from build123d import *

# Parameters (mm, degrees)
F1_W     = 279.4
F1_H     = 127
F1_W_2   = 254
F1_H_2   = 101.6
F3_DEPTH = 3.175
F2_W     = 285.75
F2_H     = 133.35
F2_W_2   = 279.4
F2_H_2   = 127
F6_DEPTH = 25.4
F7_W     = 254
F7_H     = 101.6
F7_W_2   = 247.65
F7_H_2   = 95.25
F8_DEPTH = 25.4


with BuildPart() as f3:
    # F1 (on Top) → F3 (new body)
    with BuildSketch(Plane.XY):
        Rectangle(F1_W, F1_H)
        Rectangle(F1_W_2, F1_H_2, mode=Mode.SUBTRACT)
    extrude(amount=F3_DEPTH)

    # F2 (on face) → F6 (join)
    with BuildSketch(Plane.XY):
        Rectangle(F2_W, F2_H)
        Rectangle(F2_W_2, F2_H_2, mode=Mode.SUBTRACT)
    extrude(amount=F6_DEPTH)

    # F7 (on face) → F8 (join)
    with BuildSketch(Plane.XY):
        Rectangle(F7_W, F7_H)
        Rectangle(F7_W_2, F7_H_2, mode=Mode.SUBTRACT)
    extrude(amount=F8_DEPTH)


solid = f3.part
Check sheet for the modelled part. Datum: model origin and axes. Units: mm. A direction names the side the tool comes from. Coordinates: 2 decimals unless noted, no trailing zeros. Loops run counter-clockwise (first coordinate to the right, second up) from the corner with the lowest first, then second, coordinate; pieces in that order, holes last. Notation, with made-up numbers: (23.25, 72) -> (44.25, 72) arc R18 cw to (44.25, 88) -> close; hole circle Ø1 at (-33.5, 81). An arc over 180 degrees is marked (long way). Write item = value, one per line. Start each with the question number.
1. Draft check along Y on faces 4 (the flat face through (-127, -1, 14)), 5 (the flat face through (-2, -66.675, 13)), 6 (the flat face through (142.875, -1, 13)). Enter one of: released by +Y, released by -Y, zero draft, split by the parting line, or undercut.
2. Section check A-A on z = 21.25. Record the cut outline in (x, y) (3 decimals).
3. Tool access check on faces 1 (the flat face through (139.7, -1, 14)), 2 (the flat face through (-1, 49, 25.4)), 3 (the flat face through (-2, -47.625, 13)). Record the directions out of +Z, -Z, +X, -X, +Y, -Y that give a thin tool (end or side, any length) a straight path to the whole face; none if there is none.
4. Section check B-B on y = -44.5. Record the cut outline in (x, z) (3 decimals), then the cut area to 3 significant figures.
5. Material ranges on line 1 (X direction, y = -13.5, z = 9.5) (3 decimals); line 2 (Y direction, x = -81, z = 15.5) (3 decimals); line 3 (X direction, y = -49.5, z = 21.75) (3 decimals), recorded low to high.
6. Section check C-C on x = 3.5. Record the cut outline in (y, z) (3 decimals), then the cut area to 3 significant figures.
Responses:
q1.face_4 = undercut
q1.face_5 = released by -Y
q1.face_6 = zero draft
q2.outline = (-142.875, -66.675) -> (142.875, -66.675) -> (142.875, 66.675) -> (-142.875, 66.675) -> close; (-127, -50.8) -> (127, -50.8) -> (127, 50.8) -> (-127, 50.8) -> close; hole (-139.7, -63.5) -> (139.7, -63.5) -> (139.7, 63.5) -> (-139.7, 63.5) -> close; hole (-123.825, -47.625) -> (123.825, -47.625) -> (123.825, 47.625) -> (-123.825, 47.625) -> close
q3.face_1 = +Z
q3.face_2 = +Z, +X, -X, +Y, -Y
q3.face_3 = +Z, -Z
q4.outline = (-142.875, 0) -> (-123.825, 0) -> (-123.825, 25.4) -> (-127, 25.4) -> (-127, 3.175) -> (-139.7, 3.175) -> (-139.7, 25.4) -> (-142.875, 25.4) -> close; (123.825, 0) -> (142.875, 0) -> (142.875, 25.4) -> (139.7, 25.4) -> (139.7, 3.175) -> (127, 3.175) -> (127, 25.4) -> (123.825, 25.4) -> close
q4.area = 403 mm2
q5.line_1 = -142.875 to -139.7, -127 to -123.825, 123.825 to 127, 139.7 to 142.875
q5.line_2 = -66.675 to -63.5, -50.8 to -47.625, 47.625 to 50.8, 63.5 to 66.675
q5.line_3 = -142.875 to -139.7, -127 to 127, 139.7 to 142.875
q6.outline = (-66.675, 0) -> (-47.625, 0) -> (-47.625, 25.4) -> (-50.8, 25.4) -> (-50.8, 3.175) -> (-63.5, 3.175) -> (-63.5, 25.4) -> (-66.675, 25.4) -> close; (47.625, 0) -> (66.675, 0) -> (66.675, 25.4) -> (63.5, 25.4) -> (63.5, 3.175) -> (50.8, 3.175) -> (50.8, 25.4) -> (47.625, 25.4) -> close
q6.area = 403 mm2
